Autodesk Inventor part; units mm, degrees
ref_plane "YZ Plane" through (0, 0, 0) normal (1, 0, 0) x (0, 1, 0)
ref_plane "XZ Plane" through (0, 0, 0) normal (0, 1, 0) x (-1, 0, 0)
ref_plane "XY Plane" through (0, 0, 0) normal (0, 0, 1) x (1, 0, 0)
sketch "Skizze1" plane through (0, 0, 0) normal (0, 1, 0) x (-1, 0, 0)
  line L0 (0, 0) -> (72, 0)
  line L1 (72, 0) -> (72, -72)
  line L2 (72, -72) -> (0, -72)
  line L3 (0, -72) -> (0, 0)
  dimension "d6" = 72
  dimension "STECKDOSE" = 72
extrude "Extrusion1" add sketch "Skizze1" along normal blind 5
sketch "Skizze2" plane through (0, 5, 0) normal (0, 1, 0) x (1, 0, 0)
  line L0 (-72, 72) -> (-72, 0)
  line L1 (0, 0) -> (0, 72)
  line L2 (-72, 0) -> (0, 0)
  point P0 (-8, 8)
  dimension "d23" = 8
  dimension "d24" = 8
hole "Bohrung1" at (-8, 5, -8) direction (0, -1, 0) diameter 4 end through all
pattern_linear "Rechteckige Anordnung1" count 2 spacing 56 along (-1, 0, 0) count 2 spacing 56 along (0, 0, -1) of "Bohrung1"
chamfer "Fasen1" distance 1 angle 45 4 edges at (-36, 5, 0) (-72, 5, -36) (-36, 5, -72) (0, 5, -36)
sketch "Skizze3" plane through (0, 0, 0) normal (0, -1, 0) x (1, 0, 0)
  circle A0 centre (-36, -36) radius 28
  line L0 (-72, 0) -> (0, 0)
  line L1 (-72, -72) -> (-72, 0)
  point P0 (-36, 0)
  point P1 (-72, -36)
  dimension "d28" = 56
extrude "Extrusion2" add sketch "Skizze3" along normal blind 36
sketch "Skizze4" plane through (0, 5, 0) normal (0, 1, 0) x (1, 0, 0)
  circle A0 centre (-36, 36) radius 19.5
  line L0 (0, 72) -> (-72, 72)
  line L1 (0, 0) -> (0, 72)
  point P0 (-36, 72)
  point P1 (0, 36)
  dimension "d31" = 39
extrude "Extrusion3" cut sketch "Skizze4" against normal blind 28
equation "\"d6\" = STECKDOSE"
properties part number "Steckdose" material "PC/ABS-Kunststoff"
Verification items for the finished model (mm, model axes). A direction names the side the tool comes from. Give positions to 0.01 mm unless a question says otherwise; leave off trailing zeros. Order: outer loops, then holes, each group sorted by start corner. A loop starts at its lowest first (then second) coordinate and runs counter-clockwise, first axis right, second up. Notation, with made-up numbers: M 63.25,78.25 L 95.25,78.25 A19 cw 95.25,105.25 Z; hole C 23.5,56.25 d11. An arc over 180 degrees is marked long. Return JSON: item names as keys, results as strings. Group by question number.
1) Access from +Z, -Z, +X, -X, +Y, -Y to the whole of each face (thin tool, end or side, straight path). Record for faces 1 (the face through (-51.5, 0, -59.5)), 2 (the face through (-40.227, -8.804, -16.964)), 3 (the face through (-36, -36, -36)).
2) Mould release check, pull along Z, two halves, no side actions. Record for faces 4 (the face through (-35, 2, 0)), 5 (the face through (-23.08, -17.75, -11.16)), 6 (the face through (-72, 2, -35)), 7 (the face through (-36, -23, -36)): pulls with the +Z half, pulls with the -Z half, needs draft (parallel to the pull), parting line crosses it, or undercut.
3) Section check B-B on z = -17.5. Record the cut outline in (x, y), and give its area (3 significant figures).
4) Section check A-A on z = -63. Record the cut outline in (x, y).
5) Section check D-D on x = -39. Record the cut outline in (y, z), and give its area (3 significant figures).
6) Section check C-C on y = -22. Record the cut outline in (x, z), and give its area (3 significant figures).
7) Go/stop test with flat-tipped pins: pin 1 Ø11.5 at (x, z) = (-37.5, -30) entering from +Y; pin 2 Ø1 at (x, y) = (-45, -19.5) entering from +Z; pin 3 Ø8 at (y, z) = (-6, -8.5) entering from +X. Record where each tip stops, or that it passes through.
8) Scan lines: line 1 (Z direction, x = -64, y = 3.9); line 2 (Y direction, x = -19, z = -31.5). Record each from-to range of solid material in increasing order.
Answer block:
{
 "1": {"face 1": "-Y", "face 2": "+Y", "face 3": "+Z, -Z, +X, -X, -Y"},
 "2": {"face 4": "pulls with the +Z half", "face 5": "parting line crosses it", "face 6": "needs draft", "face 7": "undercut"},
 "3": {"outline": "M -72,0 L -57.02,0 L -57.02,-36 L -14.98,-36 L -14.98,0 L 0,0 L 0,4 L -1,5 L -29.84,5 L -29.84,-23 L -42.16,-23 L -42.16,5 L -71,5 L -72,4 Z", "area": "1,530 mm^2"},
 "4": {"outline": "M -72,0 L -65.73,0 L -65.73,5 L -71,5 L -72,4 Z; M -62.27,0 L -43.42,0 L -43.42,-36 L -28.58,-36 L -28.58,0 L -9.73,0 L -9.73,5 L -62.27,5 Z; M -6.27,0 L 0,0 L 0,4 L -1,5 L -6.27,5 Z"},
 "5": {"outline": "M -36,-63.84 L 0,-63.84 L 0,-72 L 4,-72 L 5,-71 L 5,-55.27 L -23,-55.27 L -23,-16.73 L 5,-16.73 L 5,-1 L 4,0 L 0,0 L 0,-8.16 L -36,-8.16 Z", "area": "1,280 mm^2"},
 "6": {"outline": "C -36,-36 d56; hole C -36,-36 d39", "area": "1,270 mm^2"},
 "7": {"pin 1": "stops at y = -23", "pin 2": "stops at z = -9.32", "pin 3": "stops at x = -20.78"},
 "8": {"line 1": "z = -72 to -66, -62 to -10, -6 to 0", "line 2": "y = -36 to -23"}
}
